from build123d import *

# Parameters (mm, degrees)
SKETCH2_R           = 3.175
SKETCH2_R_2         = 2
SKETCH2_R_3         = 1.905
BOSS_EXTRUDE1_DEPTH = 6.35


with BuildPart() as part:
    # Sketch2 → Boss-Extrude1 (new body)
    with BuildSketch(Plane(origin=(0, 0, 0), x_dir=(1, 0, 0), z_dir=(0, 1, 0))):
        with BuildLine():
            Line((-16.51, -3.81), (-16.51, -231.775))
            Line((-16.51, -231.775), (16.51, -212.710894111))
            Line((16.51, -212.710894111), (16.51, -28.712717762))
            Line((16.51, -28.712717762), (13.335, -26.879630657))
            ThreePointArc((13.335, -26.879630657), (12.006115832, -25.385120864), (11.834308438, -23.392641284))
            Line((11.834308438, -23.392641284), (16.51, -3.81))
            ThreePointArc((16.51, -3.81), (0, 12.7), (-16.51, -3.81))
        make_face()
        with Locations(Location((0, 0, 0), (0, 0, 270))):
            Circle(SKETCH2_R, mode=Mode.SUBTRACT)
        with Locations(Location((-11.43, -219.075, 0), (0, 0, 270))):
            Circle(SKETCH2_R_2, mode=Mode.SUBTRACT)
        with Locations(Location((-11.43, -212.725, 0), (0, 0, 270))):
            Circle(SKETCH2_R_2, mode=Mode.SUBTRACT)
        with Locations(Location((-11.43, -206.375, 0), (0, 0, 270))):
            Circle(SKETCH2_R_2, mode=Mode.SUBTRACT)
        with Locations(Location((-11.43, -200.025, 0), (0, 0, 270))):
            Circle(SKETCH2_R_2, mode=Mode.SUBTRACT)
        with Locations(Location((-10.6553, -63.5, 0), (0, 0, 270))):
            Circle(SKETCH2_R_3, mode=Mode.SUBTRACT)
        with Locations(Location((12.7, -38.1, 0), (0, 0, 270))):
            Circle(SKETCH2_R_2, mode=Mode.SUBTRACT)
    extrude(amount=BOSS_EXTRUDE1_DEPTH)


solid = part.part
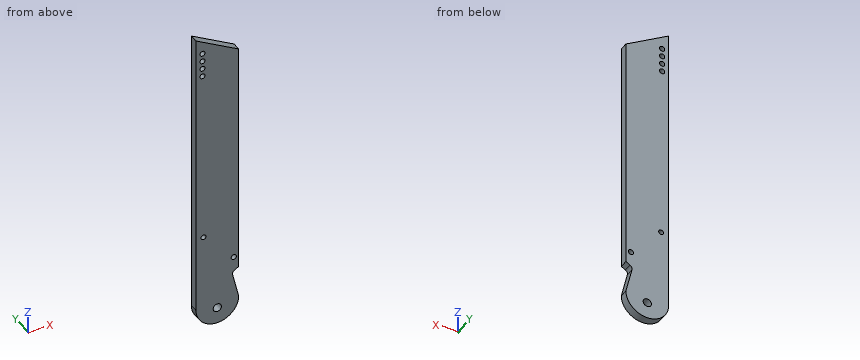
Work out the finished part from the listing and answer in its coordinate system (mm). Give positions to 0.01 mm unless a question says otherwise; leave off trailing zeros. Order: outer loops, then holes, each group sorted by start corner. A loop starts at its lowest first (then second) coordinate and runs counter-clockwise, first axis right, second up. Notation, with made-up numbers: (34.25, 61.25) -> (42.25, 61.25) arc R34 cw to (42.25, 92.25) -> close; hole circle Ø1 at (-2.5, -2.75). An arc over 180 degrees is marked (long way). Answer as a JSON object with one key per item and string values. Group by question number.
1. Section B-B on x = 0 is taken. Determine the outline of the cut face in (y, z) (3 decimals).
2. Section C-C on y = 1.25 is taken. Count the separate pieces of the cut face and the enclosed holes in it, plus the area to 3 significant figures.
3. Flat-ended cylindrical pins translate along their axes: pin 1 Ø1 at (x, y) = (11, 4.5) entering from +Z; pin 2 Ø2 at (x, z) = (8, 176.5) entering from -Y; pin 3 Ø1 at (x, y) = (9, 3.5) entering from +Z; pin 4 Ø3.5 at (x, z) = (-10.66, 63.5) entering from +Y. Find the tip coordinate at first contact, or state that the pin passes through.
4. Section A-A on z = 38.1 is taken. Determine the outline of the cut face in (x, y).
5. Consider line 1 along Z through (x, y) = (-10.5, 2.75); line 2 along X through (y, z) = (1.75, 38.1); line 3 along Z through (x, y) = (11, 3.5). Determine where each line is inside the solid, lowest interval first. Write a range as [from, to].
Result sheet:
{
 "1": {"outline": "(0, -12.7) -> (6.35, -12.7) -> (6.35, -3.175) -> (0, -3.175) -> close; (0, 3.175) -> (6.35, 3.175) -> (6.35, 222.243) -> (0, 222.243) -> close"},
 "2": {"separate pieces": "1", "enclosed holes": "7", "area": "7,470 mm^2"},
 "3": {"pin 1": "stops at z = 216.18", "pin 2": "stops at y = 0", "pin 3": "stops at z = 217.34", "pin 4": "passes through"},
 "4": {"outline": "(-16.51, 0) -> (10.7, 0) -> (10.7, 6.35) -> (-16.51, 6.35) -> close; (14.7, 0) -> (16.51, 0) -> (16.51, 6.35) -> (14.7, 6.35) -> close"},
 "5": {"line 1": "z = [-8.93, 61.6], [65.4, 198.25], [201.8, 204.6], [208.15, 210.95], [214.5, 217.3], [220.85, 228.31]", "line 2": "x = [-16.51, 10.7], [14.7, 16.51]", "line 3": "z = [-8.5, 37.05], [39.15, 215.89]"}
}
